```python
from build123d import *

# Parameters (mm, degrees)
SKETCH1_R           = 15.367
BOSS_EXTRUDE1_DEPTH = 2.794
CIRPATTERN1_COUNT   = 6
CHAMFER1_SIZE       = 1.27


with BuildPart() as part:
    # Sketch1 → Boss-Extrude1 (new body)
    with BuildSketch(Plane.XY):
        Circle(SKETCH1_R)
    extrude(amount=BOSS_EXTRUDE1_DEPTH)

    # Sketch3 → Cut-Revolve1 (revolve, cut)
    with BuildSketch(Plane(origin=(0, 0, 0), x_dir=(0, 0, -1), z_dir=(1, 0, 0))):
        with BuildLine():
            Line((-6.14045, 8.255), (-0.97155, 8.255))
            ThreePointArc((-0.97155, 8.255), (-3.556, 10.83945), (-6.14045, 8.255))
        make_face()
    cut_revolve1 = revolve(axis=Axis((0, 8.255, 6.14045), (0, 0, -1)), mode=Mode.SUBTRACT)

    # CirPattern1: Cut-Revolve1 ×6 about axis
    cirpattern1_axis = Axis((0, 0, 0), (0, 0, 1))
    for i in range(1, CIRPATTERN1_COUNT):
        add(cut_revolve1.rotate(cirpattern1_axis, i * 360 / CIRPATTERN1_COUNT), mode=Mode.SUBTRACT)

    # Chamfer1
    chamfer1_edges = [part.edges().sort_by_distance(p)[0] for p in [
        (-15.367, 0, 2.794),
    ]]
    chamfer(chamfer1_edges, length=CHAMFER1_SIZE)


solid = part.part
```
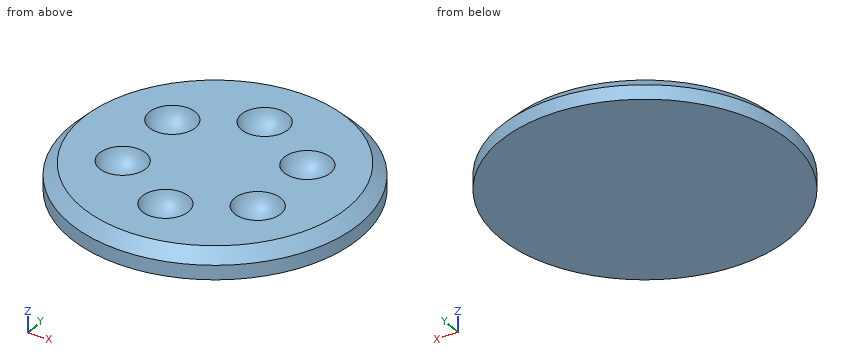
Build history of the part. All positions in model axes, mm. Give positions to 0.01 mm unless a question says otherwise; leave off trailing zeros. Loops run counter-clockwise (first coordinate to the right, second up) from the corner with the lowest first, then second, coordinate; pieces in that order, holes last.
1) Band-saw the part on B-B on y = 0. List the corners of the cut face in (x, z), then the cut area to 3 significant figures.
Values follow:
outline: (-15.37, 0) - (15.37, 0) - (15.37, 1.52) - (14.1, 2.79) - (-14.1, 2.79) - (-15.37, 1.52) - close
area: 84.3 mm2
2) Band-saw the part on A-A on x = 0. List the corners of the cut face in (y, z) (3 decimals).
Values follow:
outline: (-15.367, 0) - (15.367, 0) - (15.367, 1.524) - (14.097, 2.794) - (10.725, 2.794) arc R2.584 cw to (5.785, 2.794) - (-5.785, 2.794) arc R2.584 cw to (-10.725, 2.794) - (-14.097, 2.794) - (-15.367, 1.524) - close
3) Drop a flat-ended pin along its axis: P1, Ø1.5, axis at y = 0.5, z = 2, coming from the +X side. Give the stop position or say it passes through.
Values follow:
P1: stops at x = 15.37
4) Probe line 1 along X through (y, z) = (6, 2.15); line 2 along X through (y, z) = (-3, 2.15); line 3 along Z through (x, y) = (2, 9). List the from-to ranges inside material, lowest first.
Values follow:
line 1: x = -13.46 to -8.24, -6.06 to 6.06, 8.24 to 13.46
line 2: x = -14.43 to -9, -5.3 to 5.3, 9 to 14.43
line 3: z = 0 to 2.1
